Input: part model. Units: mm. Frame: model coordinates. A direction names the side the tool comes from. Round coordinates to 2 decimals unless told otherwise and drop trailing zeros. Loops run counter-clockwise (first coordinate to the right, second up) from the corner with the lowest first, then second, coordinate; pieces in that order, holes last. Notation, with made-up numbers: M 69.25,57.5 L 108.25,57.5 A34 ccw 108.25,92.5 Z; hole C -18.75,88 d6. An arc over 180 degrees is marked long. Use one line per item in the form item = value. Start each with the question number.
Q1. Section query C-C, the plane z = 0.5. Output: boundary loops of the cut face in (x, y).
Q2. Ray query, line 1 along Z through (x, y) = (2.5, -12.5); line 2 along X through (y, z) = (-38.5, -11.5); line 3 along Y through (x, z) = (-55.5, 15.5). Return the intervals inside material, ascending.
Q3. Access query for faces 4 (the flat face through (-77.5, -25, 0)), 5 (the flat face through (-75.5, -24, 0)). Directions: +Z, -Z, +X, -X, +Y, -Y. A direction counts if a zero-diameter tool reaches every point of the face in a straight line with its end or side. Return the directions, or none.
Q4. Section query A-A, the plane x = -60. Output: boundary loops of the cut face in (y, z).
Q5. Section query B-B, the plane y = -17. Output: boundary loops of the cut face in (x, z).
Q6. Mould query, pull axis X, two halves, no side actions, for faces 1 (the flat face through (77.5, -25, 0)), 2 (the flat face through (-1, -24, 16)), 3 (the flat face through (0, 0, 17)). Classes: pulls with the +X half, pulls with the -X half, needs draft (parallel to the pull), parting line crosses it, or undercut.
```python
from build123d import *

# Parameters (mm, degrees)
F0_W     = 155
F0_H     = 36
F1_DEPTH = 50
F2_T     = -2
F3_W     = 44
F3_H     = 26
F4_DEPTH = 25


with BuildPart() as f1:
    # F0 (on Front) → F1 (new body)
    with BuildSketch(Plane.XZ):
        Rectangle(F0_W, F0_H)
    extrude(amount=F1_DEPTH)

    # F2
    f2_openings = [f1.faces().sort_by_distance(p)[0] for p in [
        (0, 0, 0),
    ]]
    offset(amount=F2_T, openings=f2_openings)

    # F3 (on face) → F4 (cut)
    with BuildSketch(Plane.XZ.offset(50)):
        Rectangle(F3_W, F3_H)
        with Locations((-50, 0)):
            Rectangle(F3_W, F3_H)
        with Locations((50, 0)):
            Rectangle(F3_W, F3_H)
    extrude(amount=-F4_DEPTH, mode=Mode.SUBTRACT)


solid = f1.part
```
Results found:
q1.outline = M -77.5,-50 L -72,-50 L -72,-48 L -75.5,-48 L -75.5,0 L -77.5,0 Z; M -28,-50 L -22,-50 L -22,-48 L -28,-48 Z; M 22,-50 L 28,-50 L 28,-48 L 22,-48 Z; M 72,-50 L 77.5,-50 L 77.5,0 L 75.5,0 L 75.5,-48 L 72,-48 Z
q2.line_1 = -18 to -16, 16 to 18
q2.line_2 = -77.5 to -75.5, 75.5 to 77.5
q2.line_3 = -50 to -48
q3.face_4 = +Z, -Z, -X, +Y, -Y
q3.face_5 = +Y
q4.outline = M -50,-18 L 0,-18 L 0,-16 L -48,-16 L -48,-13 L -50,-13 Z; M -50,13 L -48,13 L -48,16 L 0,16 L 0,18 L -50,18 Z
q5.outline = M -77.5,-18 L 77.5,-18 L 77.5,18 L -77.5,18 Z; hole M -75.5,-16 L 75.5,-16 L 75.5,16 L -75.5,16 Z
q6.face_1 = pulls with the +X half
q6.face_2 = undercut
q6.face_3 = needs draft
